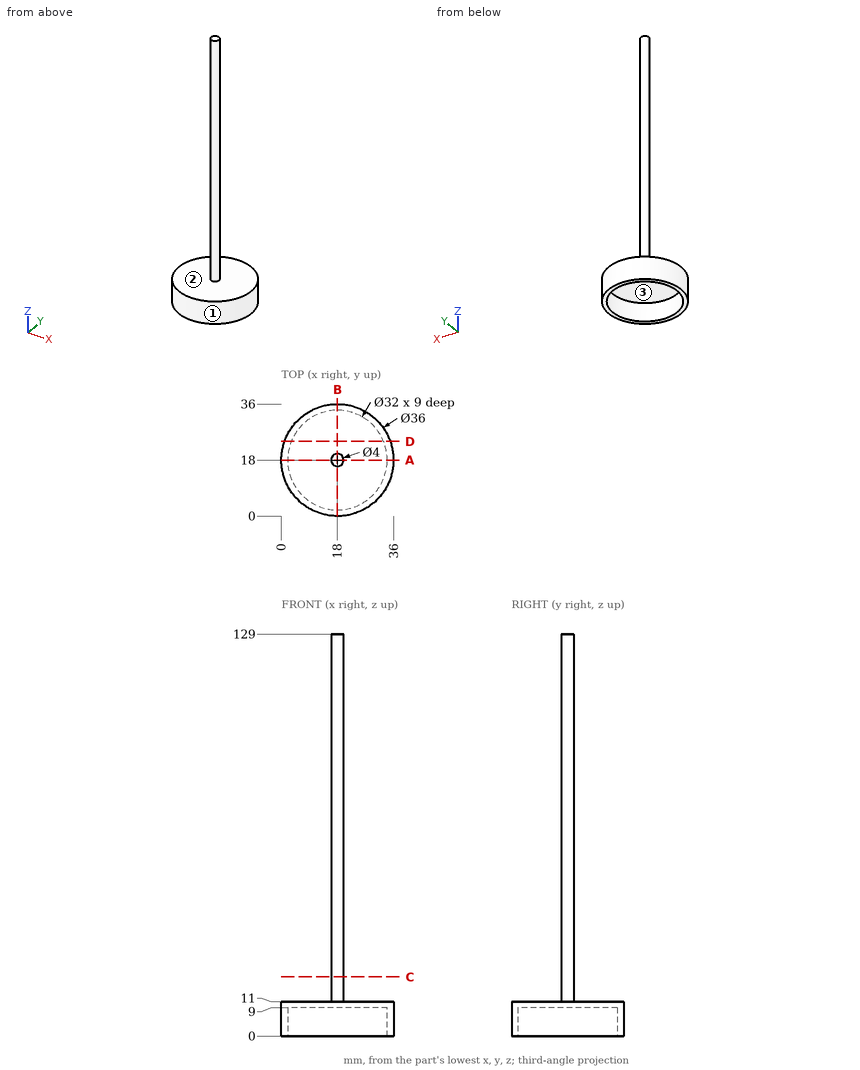
Job drawing, mm, ordinate dimensions from the low corner. One solid piece. Give positions to 0.01 mm unless a question says otherwise; leave off trailing zeros. Order: outer loops, then holes, each group sorted by start corner. A loop starts at its lowest first (then second) coordinate and runs counter-clockwise, first axis right, second up. Notation, with made-up numbers: (8, -37.5) - (39, -37.5) arc R32 ccw to (39, -6.5) - close; hole circle Ø11 at (10.5, 23.5). An arc over 180 degrees is marked (long way). One line per question, with ' | ' between items.
1. Pull direction X, two halves, no side cores. Call the marked faces 1, 2 and 3: +X half, -X half, draft (parallel to the pull), parting line (faces both ways), or undercut.
Filled in:
face 1: parting line | face 2: draft | face 3: undercut
2. Band-saw the part on A-A on y = 18. List the corners of the cut face in (x, z).
Filled in:
outline: (0, 0) - (2, 0) - (2, 9) - (34, 9) - (34, 0) - (36, 0) - (36, 11) - (20, 11) - (20, 129) - (16, 129) - (16, 11) - (0, 11) - close
3. Band-saw the part on D-D on y = 24. List the corners of the cut face in (x, z), then the cut area to 3 significant figures.
Filled in:
outline: (1.03, 0) - (3.17, 0) - (3.17, 9) - (32.83, 9) - (32.83, 0) - (34.97, 0) - (34.97, 11) - (1.03, 11) - close | area: 106 mm²
4. Drop flat-ended pins along their axis: P1, Ø1, axis at y = 17.5, z = 51.5, coming from the -X side; P2, Ø10, axis at x = 19, z = 18.5, coming from the -Y side; P3, Ø11, axis at x = 22.5, y = 11, coming from the +Z side. Give the stop position or say it passes through.
Filled in:
P1: x = 16 | P2: y = 16 | P3: z = 11
5. Drill centre lines: probe 1 along Y at (x, z) = (18, 2.5); probe 2 along Z at (x, y) = (23.5, 8); probe 3 along Z at (x, y) = (25.5, 33). Where is each one in solid material? Low to high.
Filled in:
probe 1: 0 to 2, 34 to 36 | probe 2: 9 to 11 | probe 3: 0 to 11
6. Band-saw the part on C-C on z = 19. List the corners of the cut face in (x, y).
Filled in:
outline: circle Ø4 at (18, 18)
